The figure shows three views and two pictorial views of one solid part (mm, origin at its lowest corner). Answer the questions. A direction names the side the tool comes from. Coordinates: 2 decimals unless noted, no trailing zeros. Order: outer loops, then holes, each group sorted by start corner. A loop starts at its lowest first (then second) coordinate and runs counter-clockwise, first axis right, second up. Notation, with made-up numbers: M 41,40.5 L 52,40.5 A20 cw 52,49.5 Z; hole C 55,-18 d2. An arc over 180 degrees is marked long. Use a Markdown table: item, result.
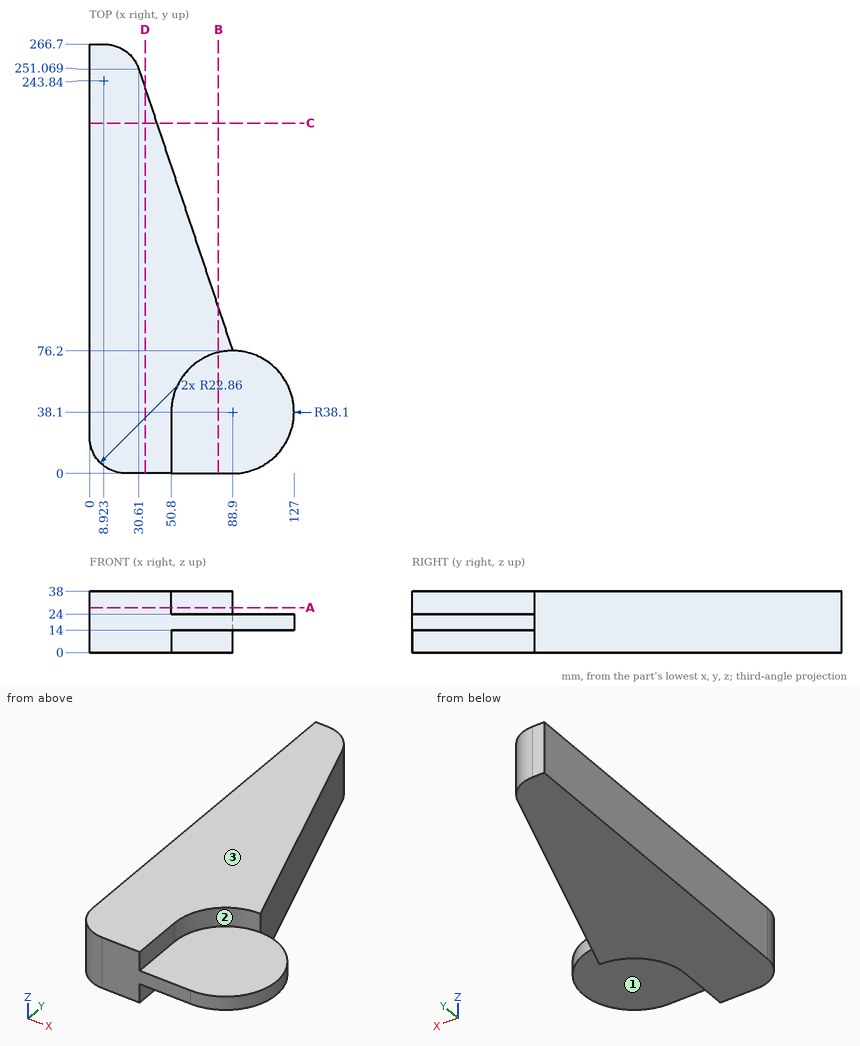
1. Section A-A on z = 28 is taken. Determine the outline of the cut face in (x, y).
Answers below:
| item | result |
|---|---|
| outline | M 0,22.86 A22.86 ccw 22.86,0 L 50.8,0 L 50.8,38.1 A38.1 cw 88.9,76.2 L 30.61,251.07 A22.86 ccw 8.92,266.7 L 0,266.7 Z |
2. Flat-ended cylindrical pins translate along their axes: P1, Ø10, axis at x = 57, z = 27, coming from the -Y side; P2, Ø4, axis at y = 26, z = 33.5, coming from the +X side; P3, Ø2, axis at x = 96, z = 12, coming from the -Y side; P4, Ø4, axis at x = 56.5, y = 43.5, coming from the -Z side. Find the tip coordinate at first contact, or state that the pin passes through.
Answers below:
| item | result |
|---|---|
| P1 | y = 0 |
| P2 | x = 50.8 |
| P3 | through |
| P4 | z = 14 |
3. For the marked faces 1, 2 and 3, determine the directions among +Z, -Z, +X, -X, +Y, -Y from which every point of the face is accessible in a straight line to the end or side of a thin tool.
Answers below:
| item | result |
|---|---|
| face 1 | -Z, +X, -Y |
| face 2 | +Z, +X, -Y |
| face 3 | +Z, +X, -X, +Y, -Y |
4. Section B-B on x = 80 is taken. Determine the outline of the cut face in (y, z), then the cut area to 3 significant figures.
Answers below:
| item | result |
|---|---|
| outline | M 0,14 L 75.15,14 L 75.15,0 L 102.9,0 L 102.9,38 L 75.15,38 L 75.15,24 L 0,24 Z |
| area | 1,810 mm² |
5. Section D-D on x = 34.5 is taken. Determine the outline of the cut face in (y, z).
Answers below:
| item | result |
|---|---|
| outline | M 0,0 L 239.4,0 L 239.4,38 L 0,38 Z |
6. Section C-C on y = 217.5 is taken. Determine the outline of the cut face in (x, z), then the cut area to 3 significant figures.
Answers below:
| item | result |
|---|---|
| outline | M 0,0 L 41.8,0 L 41.8,38 L 0,38 Z |
| area | 1,590 mm² |
7. Find the intervals of material crossed by probe 1 along Z at (x, y) = (74.5, 30); probe 2 along X at (y, z) = (31, 28); probe 3 along X at (y, z) = (40, 33.5), in increasing order.
Answers below:
| item | result |
|---|---|
| probe 1 | 14 to 24 |
| probe 2 | 0 to 50.8 |
| probe 3 | 0 to 50.85 |
